```python
from build123d import *

# Parameters (mm, degrees)
F1_DEPTH = 3


with BuildPart() as f1:
    # F0 (on Top) → F1 (new body)
    with BuildSketch(Plane.XY):
        with BuildLine():
            Line((148.364816542, 48.2066511225), (157.875381705, 51.2968210662))
            ThreePointArc((157.875381705, 51.2968210662), (97.5723518806, 134.2968210662), (0, 166))
            Line((0, 166), (0, 156))
            ThreePointArc((0, 156), (1.767766953, 155.267766953), (2.5, 153.5))
            ThreePointArc((2.5, 153.5), (1.767766953, 151.732233047), (0, 151))
            Line((0, 151), (0, 0))
            Line((0, 0), (143.6095339606, 46.6615661506))
            ThreePointArc((143.6095339606, 46.6615661506), (145.2146327654, 49.8117499273), (148.364816542, 48.2066511225))
        make_face()
        with BuildLine():
            ThreePointArc((97.5723518806, -134.2968210662), (147.9070830153, -75.3624229568), (166, 0))
            ThreePointArc((166, 0), (163.9562645388, 25.9681211967), (157.875381705, 51.2968210662))
            Line((157.875381705, 51.2968210662), (148.364816542, 48.2066511225))
            ThreePointArc((148.364816542, 48.2066511225), (148.4563961028, 47.8251947992), (148.4871752513, 47.4341086366))
            ThreePointArc((148.4871752513, 47.4341086366), (146.3782614139, 44.9648877851), (143.6095339606, 46.6615661506))
            Line((143.6095339606, 46.6615661506), (0, 0))
            Line((0, 0), (88.7555730962, -122.1615661506))
            ThreePointArc((88.7555730962, -122.1615661506), (91.3600124762, -121.9565923261), (92.7250362269, -124.1841086366))
            ThreePointArc((92.7250362269, -124.1841086366), (92.4525525374, -125.3190848859), (91.6944993576, -126.2066511225))
            Line((91.6944993576, -126.2066511225), (97.5723518806, -134.2968210662))
        make_face()
        with BuildLine():
            ThreePointArc((-97.5723518806, -134.2968210662), (0, -166), (97.5723518806, -134.2968210662))
            Line((97.5723518806, -134.2968210662), (91.6944993576, -126.2066511225))
            ThreePointArc((91.6944993576, -126.2066511225), (88.202493741, -125.6535717673), (88.7555730962, -122.1615661506))
            Line((88.7555730962, -122.1615661506), (0, 0))
            Line((0, 0), (-88.7555730962, -122.1615661506))
            ThreePointArc((-88.7555730962, -122.1615661506), (-87.9975199164, -123.0491323872), (-87.7250362269, -124.1841086366))
            ThreePointArc((-87.7250362269, -124.1841086366), (-89.0900599775, -126.411624947), (-91.6944993576, -126.2066511225))
            Line((-91.6944993576, -126.2066511225), (-97.5723518806, -134.2968210662))
        make_face()
        with BuildLine():
            ThreePointArc((-157.875381705, 51.2968210662), (-157.875381705, -51.2968210662), (-97.5723518806, -134.2968210662))
            Line((-97.5723518806, -134.2968210662), (-91.6944993576, -126.2066511225))
            ThreePointArc((-91.6944993576, -126.2066511225), (-92.2475787128, -122.7146455058), (-88.7555730962, -122.1615661506))
            Line((-88.7555730962, -122.1615661506), (0, 0))
            Line((0, 0), (-143.6095339606, 46.6615661506))
            ThreePointArc((-143.6095339606, 46.6615661506), (-146.7597177372, 45.0564673458), (-148.364816542, 48.2066511225))
            Line((-148.364816542, 48.2066511225), (-157.875381705, 51.2968210662))
        make_face()
        with BuildLine():
            Line((0, 156), (0, 166))
            ThreePointArc((0, 166), (-97.5723518806, 134.2968210662), (-157.875381705, 51.2968210662))
            Line((-157.875381705, 51.2968210662), (-148.364816542, 48.2066511225))
            ThreePointArc((-148.364816542, 48.2066511225), (-145.5960890887, 49.903329488), (-143.4871752513, 47.4341086366))
            ThreePointArc((-143.4871752513, 47.4341086366), (-143.5179543998, 47.043022474), (-143.6095339606, 46.6615661506))
            Line((-143.6095339606, 46.6615661506), (0, 0))
            Line((0, 0), (0, 151))
            ThreePointArc((0, 151), (-2.5, 153.5), (0, 156))
        make_face()
    extrude(amount=F1_DEPTH)


solid = f1.part
```
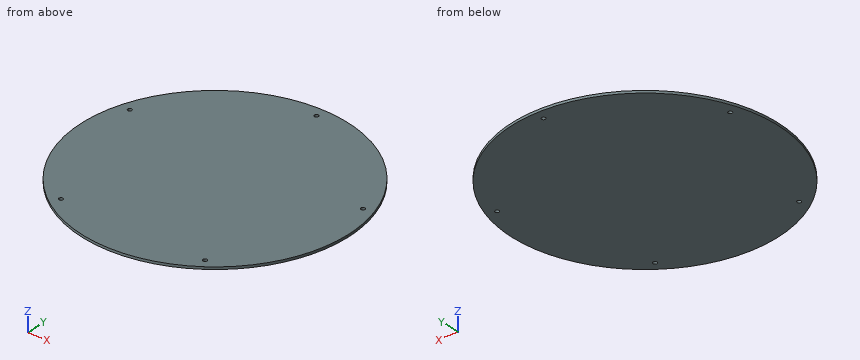
Check sheet for the modelled part. Datum: model origin and axes. Units: mm. Give positions to 0.01 mm unless a question says otherwise; leave off trailing zeros. Write each loop counter-clockwise with the first axis right and the second up, starting at its lowest first coordinate (ties: lowest second). Pieces come first, ordered by that corner, then holes.
Item 1: Cross-section at A-A (z = 0.6). Enter the section's corners in (x, y), and give its area (3 significant figures).
Item 2: Cross-section at C-C (x = 54.5). Enter the section's corners in (y, z).
Item 3: Scan lines: L1, parallel to Y at x = -144, z = 0.5; L2, parallel to Y at x = -59, z = 2.55; L3, parallel to X at y = -133, z = 2.4. Record each from-to range of solid material in increasing order.
Item 4: Gauge pin test, flat ends, axial feed: pin 1 (1 mm diameter, centred on y = 91, z = 2.5, fed in from +X); pin 2 (1 mm diameter, centred on x = -91, z = 2.5, fed in from -Y); pin 3 (1 mm diameter, centred on x = 88, z = 1, fed in from +Y). Record the tip position at first contact, or that the pin passes through.
Item 5: Cross-section at B-B (y = 123). Enter the section's corners in (x, z).
Report:
1. outline: circle Ø332 at (0, 0); hole circle Ø5 at (-145.99, 47.43); hole circle Ø5 at (-90.23, -124.18); hole circle Ø5 at (0, 153.5); hole circle Ø5 at (90.23, -124.18); hole circle Ø5 at (145.99, 47.43)
1. area: 86,500 mm2
2. outline: (-156.8, 0) - (156.8, 0) - (156.8, 3) - (-156.8, 3) - close
3. L1: y = -82.58 to 45.92, 48.95 to 82.58
3. L2: y = -155.16 to 155.16
3. L3: x = -99.33 to 99.33
4. pin 1: stops at x = 139.16
4. pin 2: stops at y = -139.16
4. pin 3: stops at y = 141.07
5. outline: (-111.48, 0) - (111.48, 0) - (111.48, 3) - (-111.48, 3) - close
